The model under review builds one solid part; all positions refer to its coordinate system, in mm. A direction names the side the tool comes from. Round coordinates to 2 decimals unless told otherwise and drop trailing zeros. Write each loop counter-clockwise with the first axis right and the second up, starting at its lowest first coordinate (ties: lowest second). Pieces come first, ordered by that corner, then holes. Notation, with made-up numbers: (-16, 25) - (35, 25) arc R15 ccw to (35, 35) - close; hole circle Ø11 at (85.5, 38.5). An arc over 180 degrees is marked (long way). Use one line per item in the form item = value.
from build123d import *

# Parameters (mm, degrees)
ESQUISSE1_W             = 10
ESQUISSE1_H             = 5
BOSS_EXTRU_1_DEPTH      = 8
ESQUISSE2_W             = 6.6
ESQUISSE2_H             = 0.8
ENL_V_MAT_EXTRU_1_DEPTH = 8
ENL_V_MAT_EXTRU_2_DEPTH = 6.5
ESQUISSE5_W             = 6
ESQUISSE5_H             = 0.5
ENL_V_MAT_EXTRU_3_DEPTH = 1
ESQUISSE6_W             = 5.6
ESQUISSE6_H             = 0.5
ENL_V_MAT_EXTRU_4_DEPTH = 3
ESQUISSE7_W             = 0.8
ESQUISSE7_H             = 1
ENL_V_MAT_EXTRU_5_DEPTH = 10
ESQUISSE8_W             = 6.8
ESQUISSE8_H             = 4.2
ENL_V_MAT_EXTRU_6_DEPTH = 1
BOSS_EXTRU_2_DEPTH      = 6.8
BOSS_EXTRU_3_DEPTH      = 2
BOSS_EXTRU_3_DEPTH_BACK = 2
ESQUISSE12_W            = 0.5
ESQUISSE12_H            = 4.2
BOSS_EXTRU_4_DEPTH      = 1
CHANFREIN1_SIZE         = 0.15
ESQUISSE13_W            = 0.45
ESQUISSE13_H            = 0.45
BOSS_EXTRU_5_DEPTH      = 3.2
BOSS_EXTRU_5_DEPTH_BACK = 5
CHANFREIN2_SIZE         = 0.1


with BuildPart() as part:
    # Esquisse1 → Boss.-Extru.1 (new body)
    with BuildSketch(Plane(origin=(0, 0, 0), x_dir=(1, 0, 0), z_dir=(0, 1, 0))):
        with Locations((5, 2.5)):
            Rectangle(ESQUISSE1_W, ESQUISSE1_H)
    extrude(amount=BOSS_EXTRU_1_DEPTH)

    # Esquisse2 → Enlèv. mat.-Extru.1 (cut)
    with BuildSketch(Plane(origin=(0, 8, 0), x_dir=(1, 0, 0), z_dir=(0, 1, 0))):
        with Locations((5, 0.4)):
            Rectangle(ESQUISSE2_W, ESQUISSE2_H)
    extrude(amount=-ENL_V_MAT_EXTRU_1_DEPTH, mode=Mode.SUBTRACT)

    # Esquisse4 → Enlèv. mat.-Extru.2 (cut)
    with BuildSketch(Plane(origin=(0, 8, 0), x_dir=(1, 0, 0), z_dir=(0, 1, 0))):
        Polygon((0.5, 0.5), (1.2, 0.5), (1.2, 1.3), (8.8, 1.3), (8.8, 0.5), (9.5, 0.5), (9.5, 4.5), (0.5, 4.5), align=None)
    extrude(amount=-ENL_V_MAT_EXTRU_2_DEPTH, mode=Mode.SUBTRACT)

    # Esquisse5 → Enlèv. mat.-Extru.3 (cut)
    with BuildSketch(Plane(origin=(0, 8, 0), x_dir=(1, 0, 0), z_dir=(0, 1, 0))):
        with Locations((5, 4.75)):
            Rectangle(ESQUISSE5_W, ESQUISSE5_H)
    extrude(amount=-ENL_V_MAT_EXTRU_3_DEPTH, mode=Mode.SUBTRACT)

    # Esquisse6 → Enlèv. mat.-Extru.4 (cut)
    with BuildSketch(Plane(origin=(0, 8, 0), x_dir=(1, 0, 0), z_dir=(0, 1, 0))):
        with Locations((5, 1.05)):
            Rectangle(ESQUISSE6_W, ESQUISSE6_H)
    extrude(amount=-ENL_V_MAT_EXTRU_4_DEPTH, mode=Mode.SUBTRACT)

    # Esquisse7 → Enlèv. mat.-Extru.5 (cut)
    with BuildSketch(Plane(origin=(10, 0, 0), x_dir=(0, 0, -1), z_dir=(1, 0, 0))):
        with Locations((0.4, 0.5)):
            Rectangle(ESQUISSE7_W, ESQUISSE7_H)
    extrude(amount=-ENL_V_MAT_EXTRU_5_DEPTH, mode=Mode.SUBTRACT)

    # Esquisse8 → Enlèv. mat.-Extru.6 (cut)
    with BuildSketch(Plane.XZ):
        with Locations((5, -2.9)):
            Rectangle(ESQUISSE8_W, ESQUISSE8_H)
    extrude(amount=-ENL_V_MAT_EXTRU_6_DEPTH, mode=Mode.SUBTRACT)

    # Esquisse9 → Boss.-Extru.2 (add)
    with BuildSketch(Plane(origin=(1.6, 0, 0), x_dir=(0, 0, -1), z_dir=(1, 0, 0))):
        Polygon((4.7, 1), (3.9, 0.2), (1.9, 0.2), (1.1, 1), align=None)
    extrude(amount=BOSS_EXTRU_2_DEPTH)

    # Esquisse11 → Boss.-Extru.3 (add, two sides)
    with BuildSketch(Plane(origin=(5, 0, 0), x_dir=(0, 0, -1), z_dir=(1, 0, 0))) as boss_extru_3_sk:
        Polygon((0.8, 5), (0.1, 3.4), (0.8, 3.4), align=None)
    extrude(amount=BOSS_EXTRU_3_DEPTH)
    extrude(boss_extru_3_sk.sketch, amount=-BOSS_EXTRU_3_DEPTH_BACK)

    # Esquisse12 → Boss.-Extru.4 (add)
    with BuildSketch(Plane(origin=(0, 1, 0), x_dir=(1, 0, 0), z_dir=(0, 1, 0))):
        with Locations((5, 2.9)):
            Rectangle(ESQUISSE12_W, ESQUISSE12_H)
        with Locations((3.175, 2.9)):
            Rectangle(ESQUISSE12_W, ESQUISSE12_H)
        with Locations((6.825, 2.9)):
            Rectangle(ESQUISSE12_W, ESQUISSE12_H)
    extrude(amount=-BOSS_EXTRU_4_DEPTH)

    # Chanfrein1
    chanfrein1_edges = [part.edges().sort_by_distance(p)[0] for p in [
        (2.2, 8, -1.05),
        (7.8, 8, -1.05),
    ]]
    chamfer(chanfrein1_edges, length=CHANFREIN1_SIZE)

    # Esquisse13 → Boss.-Extru.5 (add, two sides)
    with BuildSketch(Plane.XZ.offset(-0.2)) as boss_extru_5_sk:
        with Locations((8, -2.9)):
            Rectangle(ESQUISSE13_W, ESQUISSE13_H)
        with Locations((2, -2.9)):
            Rectangle(ESQUISSE13_W, ESQUISSE13_H)
        with Locations((4, -2.9)):
            Rectangle(ESQUISSE13_W, ESQUISSE13_H)
        with Locations((6, -2.9)):
            Rectangle(ESQUISSE13_W, ESQUISSE13_H)
    extrude(amount=BOSS_EXTRU_5_DEPTH)
    extrude(boss_extru_5_sk.sketch, amount=-BOSS_EXTRU_5_DEPTH_BACK)

    # Chanfrein2
    chanfrein2_edges = [part.edges().sort_by_distance(p)[0] for p in [
        (2.225, 5.2, -2.9),
        (2, 5.2, -3.125),
        (1.775, 5.2, -2.9),
        (2, 5.2, -2.675),
        (2.225, -3, -2.9),
        (2, -3, -2.675),
        (1.775, -3, -2.9),
        (2, -3, -3.125),
        (4.225, 5.2, -2.9),
        (4, 5.2, -3.125),
        (3.775, 5.2, -2.9),
        (4, 5.2, -2.675),
        (4.225, -3, -2.9),
        (4, -3, -2.675),
        (3.775, -3, -2.9),
        (4, -3, -3.125),
        (7.775, 5.2, -2.9),
        (8, 5.2, -2.675),
        (8.225, 5.2, -2.9),
        (8, 5.2, -3.125),
        (7.775, -3, -2.9),
        (8, -3, -3.125),
        (8.225, -3, -2.9),
        (8, -3, -2.675),
        (6, 5.2, -2.675),
        (6.225, 5.2, -2.9),
        (6, 5.2, -3.125),
        (5.775, 5.2, -2.9),
        (6, -3, -2.675),
        (5.775, -3, -2.9),
        (6, -3, -3.125),
        (6.225, -3, -2.9),
    ]]
    chamfer(chanfrein2_edges, length=CHANFREIN2_SIZE)


solid = part.part
(1) Add section C-C on y = -1.25. Write out the cut boundary in (x, z) (3 decimals), then the cut area to 3 significant figures.
Geometry results:
outline = (1.775, -3.125) - (2.225, -3.125) - (2.225, -2.675) - (1.775, -2.675) - close; (3.775, -3.125) - (4.225, -3.125) - (4.225, -2.675) - (3.775, -2.675) - close; (5.775, -3.125) - (6.225, -3.125) - (6.225, -2.675) - (5.775, -2.675) - close; (7.775, -3.125) - (8.225, -3.125) - (8.225, -2.675) - (7.775, -2.675) - close
area = 0.810 mm2
(2) Add section D-D on y = 6.5. Write out the cut boundary in (x, z), then the cut area to 3 significant figures.
Geometry results:
outline = (0, -5) - (10, -5) - (10, 0) - (8.3, 0) - (8.3, -0.8) - (7.8, -0.8) - (7.8, -1.3) - (8.8, -1.3) - (8.8, -0.5) - (9.5, -0.5) - (9.5, -4.5) - (0.5, -4.5) - (0.5, -0.5) - (1.2, -0.5) - (1.2, -1.3) - (2.2, -1.3) - (2.2, -0.8) - (1.7, -0.8) - (1.7, 0) - (0, 0) - close
area = 12.0 mm2
(3) Add section A-A on z = -2.5. Write out the cut boundary in (x, y) (3 decimals).
Geometry results:
outline = (0, 0) - (1.6, 0) - (1.6, 0.2) - (2.925, 0.2) - (2.925, 0) - (3.425, 0) - (3.425, 0.2) - (4.75, 0.2) - (4.75, 0) - (5.25, 0) - (5.25, 0.2) - (6.575, 0.2) - (6.575, 0) - (7.075, 0) - (7.075, 0.2) - (8.4, 0.2) - (8.4, 0) - (10, 0) - (10, 8) - (9.5, 8) - (9.5, 1.5) - (0.5, 1.5) - (0.5, 8) - (0, 8) - close
(4) Machinability: for faces 1 (the flat face through (5, 5, -4.5)), 2 (the flat face through (4.1, 0.6, -4.3)), 3 (the flat face through (0.8, 0.5, -0.8)), which of the approach directions +Z, -Z, +X, -X, +Y, -Y give a long, thin tool a straight path to every point of the face, cutting with its end or side? Answer none if there is none.
Geometry results:
face_1 = +Y
face_2 = -Z, -Y
face_3 = +Z, +X, -X, -Y
(5) The part is to be moulded in two halves that separate along X. For faces 4 (the flat face through (10, 4, -2)), 5 (the flat face through (9.2, 0.5, -0.8)), 6 (the flat face through (5, 1.5, -3)), 7 (the flat face through (5.6, 0.2, -2.9)), say which applies: +X half, -X half, draft (parallel to the pull), parting line (faces both ways), or undercut.
Geometry results:
face_4 = +X half
face_5 = draft
face_6 = undercut
face_7 = undercut
(6) To check wall thickness, follow L1, parallel to X at y = 1.75, z = -2.9 (3 decimals); L2, parallel to X at y = 0.75, z = -4.55 (3 decimals); L3, parallel to X at y = 7, z = -2.75. State the ranges of each line that lie inside material, in increasing order.
Geometry results:
L1 = 0 to 0.5, 1.775 to 2.225, 3.775 to 4.225, 5.775 to 6.225, 7.775 to 8.225, 9.5 to 10
L2 = 0 to 1.6, 2.925 to 3.425, 4.75 to 5.25, 6.575 to 7.075, 8.4 to 10
L3 = 0 to 0.5, 9.5 to 10
(7) Insertion check: P1, Ø2, axis at x = 6, y = 2, coming from the +Z side; P2, Ø3, axis at x = 5.5, y = 3.5, coming from the +Z side; P3, Ø1.5, axis at x = 7.5, z = -4, coming from the -Y side. Each pin has a flat end and moves straight along its axis. Give the tip position at first contact, or say it passes through.
Geometry results:
P1 = -0.8
P2 = -0.1
P3 = 0
(8) Add section B-B on x = 5.5. Write out the cut boundary in (y, z), then the cut area to 3 significant figures.
Geometry results:
outline = (0.2, -3.9) - (1, -4.7) - (1, -5) - (7, -5) - (7, -4.5) - (1.5, -4.5) - (1.5, -1.3) - (5, -1.3) - (5, -0.8) - (3.4, -0.1) - (3.4, -0.8) - (1, -0.8) - (1, -1.1) - (0.2, -1.9) - close
area = 9.40 mm2
